Read the model definition and answer for the solid it produces. Units are mm, in the model's axes. Give positions to 0.01 mm unless a question says otherwise; leave off trailing zeros. Loops run counter-clockwise (first coordinate to the right, second up) from the corner with the lowest first, then second, coordinate; pieces in that order, holes last. Notation, with made-up numbers: M 58,15 L 99,15 A8 ccw 99,19 Z; hole C 5,24.25 d7. An arc over 180 degrees is marked long. Return JSON: item names as keys, results as strings. Group by question number.
```python
from build123d import *

# Parameters (mm, degrees)
F1_DEPTH = 165.1
F3_DEPTH = 6.096
F4_R     = 2.286
F5_DEPTH = 25.4


with BuildPart() as f1:
    # F0 (on Front) → F1 (new body)
    with BuildSketch(Plane.XZ):
        Polygon((-88.9, 12.7), (-88.9, 0), (88.9, 0), (88.9, 6.35), (88.9, 12.7), (82.55, 12.7), (82.55, 6.35), (69.85, 6.35), (69.85, 12.7), (57.15, 12.7), (57.15, 6.35), (44.45, 6.35), (44.45, 12.7), (31.75, 12.7), (31.75, 6.35), (19.05, 6.35), (19.05, 12.7), (6.35, 12.7), (6.35, 6.35), (-6.35, 6.35), (-6.35, 12.7), (-19.05, 12.7), (-19.05, 6.35), (-31.75, 6.35), (-31.75, 12.7), (-44.45, 12.7), (-44.45, 6.35), (-57.15, 6.35), (-57.15, 12.7), (-69.85, 12.7), (-69.85, 6.35), (-82.55, 6.35), (-82.55, 12.7), align=None)
    extrude(amount=F1_DEPTH)

    # F2 (on face) → F3 (cut)
    with BuildSketch(Plane(origin=(0, 0, 0), x_dir=(1, 0, 0), z_dir=(0, 0, -1))):
        with BuildLine():
            Line((85.725, 126.746), (88.9, 126.746))
            Line((88.9, 126.746), (88.9, 139.7))
            Line((88.9, 139.7), (85.725, 139.7))
            ThreePointArc((85.725, 139.7), (79.248, 133.223), (85.725, 126.746))
        make_face()
        with BuildLine():
            Line((88.9, 25.4), (88.9, 38.354))
            Line((88.9, 38.354), (85.725, 38.354))
            ThreePointArc((85.725, 38.354), (79.248, 31.877), (85.725, 25.4))
            Line((85.725, 25.4), (88.9, 25.4))
        make_face()
        with BuildLine():
            Line((-88.9, 139.7), (-88.9, 126.746))
            Line((-88.9, 126.746), (-85.725, 126.746))
            ThreePointArc((-85.725, 126.746), (-79.248, 133.223), (-85.725, 139.7))
            Line((-85.725, 139.7), (-88.9, 139.7))
        make_face()
        with BuildLine():
            Line((-85.725, 38.354), (-88.9, 38.354))
            Line((-88.9, 38.354), (-88.9, 25.4))
            Line((-88.9, 25.4), (-85.725, 25.4))
            ThreePointArc((-85.725, 25.4), (-79.248, 31.877), (-85.725, 38.354))
        make_face()
    extrude(amount=-F3_DEPTH, mode=Mode.SUBTRACT)

    # F4 (on face) → F5 (cut)
    with BuildSketch(Plane(origin=(0, 0, 0), x_dir=(1, 0, 0), z_dir=(0, 0, -1))):
        with Locations((-85.725, 133.223)):
            Circle(F4_R)
        with Locations((85.725, 133.223)):
            Circle(F4_R)
        with Locations((85.725, 31.877)):
            Circle(F4_R)
        with Locations((-85.725, 31.877)):
            Circle(F4_R)
    extrude(amount=-F5_DEPTH, mode=Mode.SUBTRACT)


solid = f1.part
```
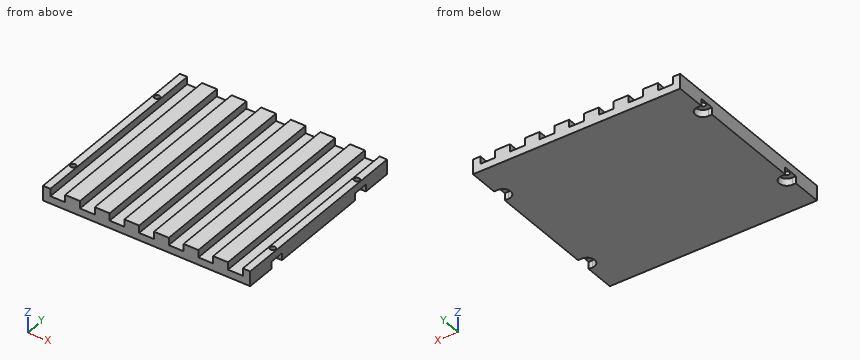
1. Find section C-C (z = 9.5). State how many separate pieces and enclosed holes the cut face has, and give its area (3 significant figures).
2. Straight lines are drawn through the part: line 1 along Z through (x, y) = (76, -55); line 2 along X through (y, z) = (-27, 5). For each, find the intervals that lie inside material, in ascending order.
3. Find section B-B (x = -1). Write down the section's boundary in (y, z).
4. Flat-ended cylindrical pins translate along their axes: P1, Ø1.5, axis at x = 4.5, z = 7.5, coming from the -Y side; P2, Ø5.5, axis at x = -85.725, y = -31.877, coming from the -Z side; P3, Ø6, axis at x = -19.5, y = -121, coming from the -Z side; P4, Ø10, axis at x = -25.5, y = -51.5, coming from the +Z side. Find the tip coordinate at first contact, or state that the pin passes through.
Result:
{
 "1": {"separate pieces": "8", "enclosed holes": "4", "area": "14,600 mm2"},
 "2": {"line 1": "z = 0 to 6.35", "line 2": "x = -81.46 to 81.46"},
 "3": {"outline": "M -165.1,0 L 0,0 L 0,6.35 L -165.1,6.35 Z"},
 "4": {"P1": "passes through", "P2": "stops at z = 6.1", "P3": "stops at z = 0", "P4": "stops at z = 6.35"}
}
